The listing builds one solid part. Answer for the finished solid, in the listing's coordinates (mm). Coordinates: 2 decimals unless noted, no trailing zeros. Order: outer loops, then holes, each group sorted by start corner. A loop starts at its lowest first (then second) coordinate and runs counter-clockwise, first axis right, second up. Notation, with made-up numbers: (55.25, 35) - (78.25, 35) arc R16 cw to (78.25, 52) - close; hole circle Ø2 at (-24.5, -40). An arc over 180 degrees is marked (long way). One line per item, written item: value. Start each with the question number.
Autodesk Inventor part; units mm, degrees
ref_plane "YZ Plane" through (0, 0, 0) normal (1, 0, 0) x (0, 1, 0)
ref_plane "XZ Plane" through (0, 0, 0) normal (0, 1, 0) x (-1, 0, 0)
ref_plane "XY Plane" through (0, 0, 0) normal (0, 0, 1) x (1, 0, 0)
sketch "Sketch1" plane through (0, 0, 0) normal (0, 0, 1) x (1, 0, 0)
  line L0 (-31.75, -21.2471) -> (-28.8544, -21.2471)
  line L1 (-28.8544, -21.2471) -> (-28.8544, -22.5171)
  line L2 (-28.8544, -22.5171) -> (28.8544, -22.5171)
  line L3 (28.8544, -22.5171) -> (28.8544, -21.2471)
  line L4 (28.8544, -21.2471) -> (31.75, -21.2471)
  line L5 (31.75, -21.2471) -> (31.75, -14.3129)
  line L6 (31.75, -14.3129) -> (28.8544, -14.3129)
  line L7 (28.8544, -14.3129) -> (28.8544, 14.3129)
  line L8 (28.8544, 14.3129) -> (31.75, 14.3129)
  line L9 (31.75, 14.3129) -> (31.75, 21.2471)
  line L10 (31.75, 21.2471) -> (28.8544, 21.2471)
  line L11 (28.8544, 21.2471) -> (28.8544, 22.5171)
  line L12 (28.8544, 22.5171) -> (-28.8544, 22.5171)
  line L13 (-28.8544, 22.5171) -> (-28.8544, 21.2471)
  line L14 (-28.8544, 21.2471) -> (-31.75, 21.2471)
  line L15 (-31.75, 21.2471) -> (-31.75, 14.3129)
  line L16 (-31.75, 14.3129) -> (-28.8544, 14.3129)
  line L17 (-28.8544, 14.3129) -> (-28.8544, -14.3129)
  line L18 (-28.8544, -14.3129) -> (-31.75, -14.3129)
  line L19 (-31.75, -14.3129) -> (-31.75, -21.2471)
  line L20 (18.415, -6.35) -> (23.6347, -6.35)
  line L21 (23.6347, -6.35) -> (23.6347, 6.35)
  line L22 (23.6347, 6.35) -> (18.415, 6.35)
  line L23 (18.415, 6.35) -> (18.415, 13.0429)
  line L24 (18.415, 13.0429) -> (15.875, 15.5829)
  line L25 (15.875, 15.5829) -> (-15.875, 15.5829)
  line L26 (-15.875, 15.5829) -> (-18.415, 13.0429)
  line L27 (-18.415, 13.0429) -> (-18.415, 6.35)
  line L28 (-18.415, 6.35) -> (-23.6347, 6.35)
  line L29 (-23.6347, 6.35) -> (-23.6347, -6.35)
  line L30 (-23.6347, -6.35) -> (-18.415, -6.35)
  line L31 (-18.415, -6.35) -> (-18.415, -13.0429)
  line L32 (-18.415, -13.0429) -> (-15.875, -15.5829)
  line L33 (-15.875, -15.5829) -> (15.875, -15.5829)
  line L34 (15.875, -15.5829) -> (18.415, -13.0429)
  line L35 (18.415, -13.0429) -> (18.415, -6.35)
  circle A0 centre (18.4151, -17.7801) radius 1.7526
  circle A1 centre (-18.415, 17.78) radius 1.7526
  circle A2 centre (-18.415, -17.78) radius 1.7526
  circle A3 centre (18.415, 17.78) radius 1.7526
extrude "Extrusion1" add sketch "Sketch1" along normal blind 2.8956
properties part number "pcb_mount" material "Polycarbonate, Clear"
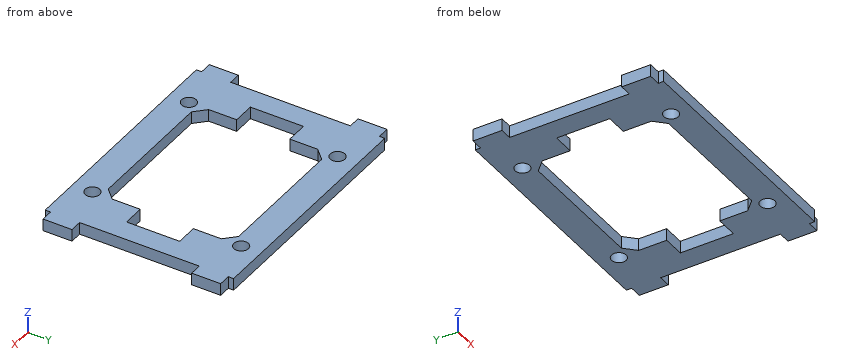
(1) The part is cut by section A-A on y = 17.78. Determine the outline of the cut face in (x, z).
(2) Consider probe 1 along Y at (x, z) = (-18.5, 1.55); probe 2 along Y at (x, z) = (23.5, 1.95); probe 3 along Y at (x, z) = (1, 1). Determine where each line is inside the solid, lowest interval first.
(3) The part is cut by section C-C on y = -3. Determine the outline of the cut face in (x, z).
(4) The part is cut by section D-D on z = 1.4. Count the separate pieces of the cut face and the enclosed holes in it, plus the area to 3 significant figures.
(5) The part is cut by section B-B on x = 3.5. Determine the outline of the cut face in (y, z), plus the area to 3 significant figures.
(6) Flat-ended cylindrical pins translate along their axes: pin 1 Ø0.6 at (y, z) = (21.5, 1) entering from +X; pin 2 Ø0.9 at (y, z) = (8.5, 2) entering from -X; pin 3 Ø3 at (x, y) = (18.42, -17.78) entering from +Z; pin 4 Ø1.4 at (y, z) = (-10.5, 2) entering from +X. Find the tip coordinate at first contact, or state that the pin passes through.
Completed:
1. outline: (-31.75, 0) - (-20.17, 0) - (-20.17, 2.9) - (-31.75, 2.9) - close; (-16.66, 0) - (16.66, 0) - (16.66, 2.9) - (-16.66, 2.9) - close; (20.17, 0) - (31.75, 0) - (31.75, 2.9) - (20.17, 2.9) - close
2. probe 1: y = -22.52 to -19.53, -16.03 to -6.35, 6.35 to 16.03, 19.53 to 22.52
2. probe 2: y = -22.52 to -6.35, 6.35 to 22.52
2. probe 3: y = -22.52 to -15.58, 15.58 to 22.52
3. outline: (-28.85, 0) - (-23.63, 0) - (-23.63, 2.9) - (-28.85, 2.9) - close; (23.63, 0) - (28.85, 0) - (28.85, 2.9) - (23.63, 2.9) - close
4. separate pieces: 1
4. enclosed holes: 5
4. area: 1,370 mm2
5. outline: (-22.52, 0) - (-15.58, 0) - (-15.58, 2.9) - (-22.52, 2.9) - close; (15.58, 0) - (22.52, 0) - (22.52, 2.9) - (15.58, 2.9) - close
5. area: 40.2 mm2
6. pin 1: stops at x = 31.75
6. pin 2: stops at x = -28.85
6. pin 3: passes through
6. pin 4: stops at x = 28.85
